Drawing for the job (mm, zero at the part's lowest x, y, z). Round coordinates to 2 decimals unless told otherwise and drop trailing zeros. Write each loop counter-clockwise with the first axis right and the second up, starting at its lowest first coordinate (ties: lowest second). Pieces come first, ordered by that corner, then holes. Notation, with made-up numbers: (86, -39.5) -> (142, -39.5) arc R25 ccw to (142, -3.5) -> close; hole circle Ø8 at (78.5, 76). An arc over 180 degrees is marked (long way). One line per question, with ' | ' between items.
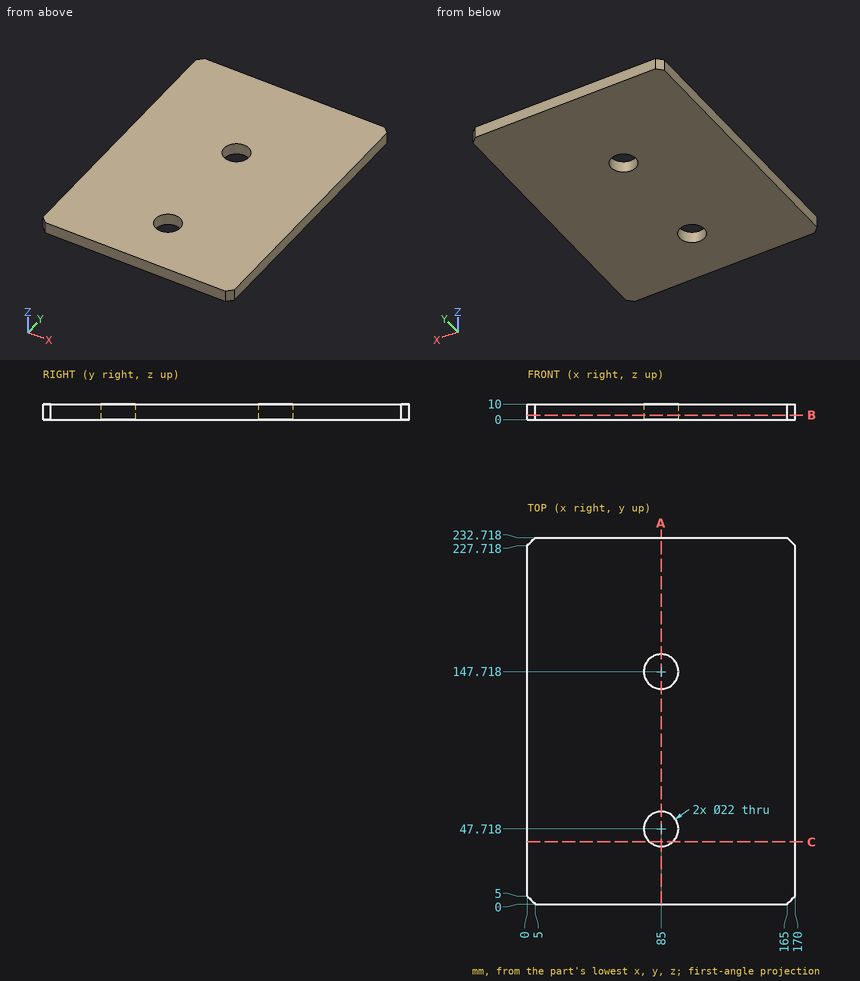
(1) Slice it at C-C (y = 39.5). Write the cut outline in (x, z), then the cut area to 3 significant figures.
Calculated:
outline: (0, 0) -> (77.69, 0) -> (77.69, 10) -> (0, 10) -> close; (92.31, 0) -> (170, 0) -> (170, 10) -> (92.31, 10) -> close | area: 1,550 mm2
(2) Slice it at B-B (z = 3). Write the cut outline in (x, y), then the cut area to 3 significant figures.
Calculated:
outline: (0, 5) -> (5, 0) -> (165, 0) -> (170, 5) -> (170, 227.72) -> (165, 232.72) -> (5, 232.72) -> (0, 227.72) -> close; hole circle Ø22 at (85, 47.72); hole circle Ø22 at (85, 147.72) | area: 38,800 mm2
(3) Slice it at A-A (x = 85). Write the cut outline in (y, z).
Calculated:
outline: (0, 0) -> (36.72, 0) -> (36.72, 10) -> (0, 10) -> close; (58.72, 0) -> (136.72, 0) -> (136.72, 10) -> (58.72, 10) -> close; (158.72, 0) -> (232.72, 0) -> (232.72, 10) -> (158.72, 10) -> close
(4) Wall check: line 1 (Y direction, x = 85, z = 7); line 2 (Y direction, x = 78.5, z = 8.25); line 3 (X direction, y = 156.5, z = 8.25). Give the ranges that are in metal, low to high. Write a range as from..to.
Calculated:
line 1: 0..36.72, 58.72..136.72, 158.72..232.72 | line 2: 0..38.84, 56.59..138.84, 156.59..232.72 | line 3: 0..78.38, 91.62..170
(5) Drop a flat-ended pin along its axis: pin 1 (5 mm diameter, centred on x = 125.5, y = 79, fed in from -Z). Give the stop position or say it passes through.
Calculated:
pin 1: z = 0
